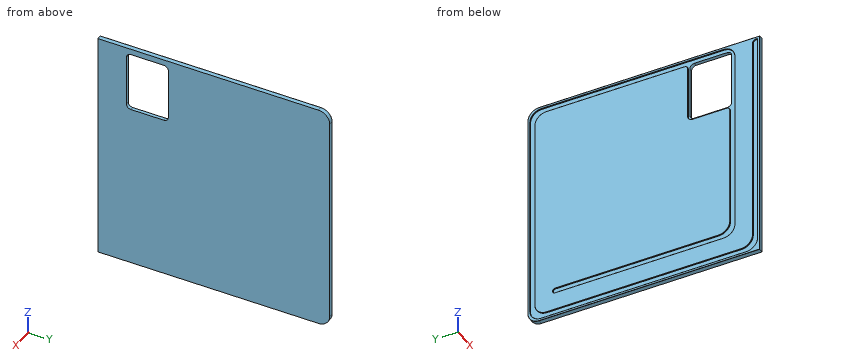
```python
from build123d import *

# Parameters (mm, degrees)
BOSS_EXTRUDE1_DEPTH = 4
CUT_EXTRUDE3_START  = -4
CUT_EXTRUDE3_DEPTH  = 1
FILLET1_R           = 0.2
CUT_EXTRUDE4_REACH  = 146.305


with BuildPart() as part:
    # Sketch1 → Boss-Extrude1 (new body)
    with BuildSketch(Plane(origin=(0, 0, 0), x_dir=(0, 0, -1), z_dir=(1, 0, 0))):
        with BuildLine():
            Line((-102, -102), (102, -102))
            Line((102, -102), (102, 92))
            ThreePointArc((102, 92), (99.071067812, 99.071067812), (92, 102))
            Line((92, 102), (-92, 102))
            ThreePointArc((-92, 102), (-99.071067812, 99.071067812), (-102, 92))
            Line((-102, 92), (-102, -102))
        make_face()
    extrude(amount=BOSS_EXTRUDE1_DEPTH)

    # Sketch2 → Cut-Extrude3 (cut)
    with BuildSketch(Plane(origin=(4, 0, 0), x_dir=(0, 0, -1), z_dir=(1, 0, 0)).offset(CUT_EXTRUDE3_START)):
        with BuildLine():
            Line((-100.1, 90.3), (-100.1, -70.3))
            ThreePointArc((-100.1, -70.3), (-97.229646456, -77.229646456), (-90.3, -80.1))
            Line((-90.3, -80.1), (70.3, -80.1))
            ThreePointArc((70.3, -80.1), (77.229646456, -77.229646456), (80.1, -70.3))
            Line((80.1, -70.3), (80.1, 78))
            ThreePointArc((80.1, 78), (78, 80.1), (75.9, 78))
            Line((75.9, 78), (75.9, -65.7))
            ThreePointArc((75.9, -65.7), (72.912489168, -72.912489168), (65.7, -75.9))
            Line((65.7, -75.9), (-40.2, -75.9))
            ThreePointArc((-40.2, -75.9), (-42.321320344, -75.021320344), (-43.2, -72.9))
            Line((-43.2, -72.9), (-43.2, -42.8))
            ThreePointArc((-43.2, -42.8), (-44.371572875, -39.971572875), (-47.2, -38.8))
            Line((-47.2, -38.8), (-92.9, -38.8))
            ThreePointArc((-92.9, -38.8), (-95.021320344, -37.921320344), (-95.9, -35.8))
            Line((-95.9, -35.8), (-95.9, 85.7))
            ThreePointArc((-95.9, 85.7), (-92.912489168, 92.912489168), (-85.7, 95.9))
            Line((-85.7, 95.9), (85.7, 95.9))
            ThreePointArc((85.7, 95.9), (92.912489168, 92.912489168), (95.9, 85.7))
            Line((95.9, 85.7), (95.9, -85.7))
            ThreePointArc((95.9, -85.7), (92.912489168, -92.912489168), (85.7, -95.9))
            Line((85.7, -95.9), (-97.3, -95.9))
            ThreePointArc((-97.3, -95.9), (-99.279898987, -96.720101013), (-100.1, -98.7))
            Line((-100.1, -98.7), (-100.1, -100.1))
            Line((-100.1, -100.1), (90.3, -100.1))
            ThreePointArc((90.3, -100.1), (97.229646456, -97.229646456), (100.1, -90.3))
            Line((100.1, -90.3), (100.1, 90.3))
            ThreePointArc((100.1, 90.3), (97.229646456, 97.229646456), (90.3, 100.1))
            Line((90.3, 100.1), (-90.3, 100.1))
            ThreePointArc((-90.3, 100.1), (-97.229646456, 97.229646456), (-100.1, 90.3))
        make_face()
        with BuildLine():
            Line((-90.9, -75.9), (-48.4, -75.9))
            ThreePointArc((-48.4, -75.9), (-46.278679656, -75.021320344), (-45.4, -72.9))
            Line((-45.4, -72.9), (-45.4, -65.9))
            Line((-45.4, -65.9), (-46.4, -65.9))
            Line((-46.4, -65.9), (-46.4, -64.4))
            Line((-46.4, -64.4), (-45.4, -64.4))
            Line((-45.4, -64.4), (-45.4, -62.5))
            Line((-45.4, -62.5), (-46.4, -62.5))
            Line((-46.4, -62.5), (-46.4, -61))
            Line((-46.4, -61), (-45.4, -61))
            Line((-45.4, -61), (-45.4, -45))
            ThreePointArc((-45.4, -45), (-46.571572875, -42.171572875), (-49.4, -41))
            Line((-49.4, -41), (-92.9, -41))
            ThreePointArc((-92.9, -41), (-95.021320344, -41.878679656), (-95.9, -44))
            Line((-95.9, -44), (-95.9, -61))
            Line((-95.9, -61), (-94.9, -61))
            Line((-94.9, -61), (-94.9, -62.5))
            Line((-94.9, -62.5), (-95.9, -62.5))
            Line((-95.9, -62.5), (-95.9, -64.4))
            Line((-95.9, -64.4), (-94.9, -64.4))
            Line((-94.9, -64.4), (-94.9, -65.9))
            Line((-94.9, -65.9), (-95.9, -65.9))
            Line((-95.9, -65.9), (-95.9, -70.9))
            ThreePointArc((-95.9, -70.9), (-94.435533906, -74.435533906), (-90.9, -75.9))
        make_face(mode=Mode.SUBTRACT)
    extrude(amount=CUT_EXTRUDE3_DEPTH, mode=Mode.SUBTRACT)

    # Fillet1
    fillet1_edges = [part.edges().sort_by_distance(p)[0] for p in [
        (0, -72.912489168, -72.912489168),
        (0, -75.021320344, 42.321320344),
        (0, -37.921320344, 95.021320344),
        (0, 92.912489168, 92.912489168),
        (0, 92.912489168, -92.912489168),
        (0, -92.912489168, -92.912489168),
        (0, -96.720101013, 99.279898987),
        (0, -95.9, 5.8),
        (0, 0, -95.9),
        (0, 95.9, 0),
        (0, 24.95, 95.9),
        (0, -38.8, 70.05),
        (0, -39.971572875, 44.371572875),
        (0, -57.85, 43.2),
        (0, -75.9, -12.75),
        (0, 6.15, -75.9),
        (0, 80.1, -78),
        (0, 3.85, -80.1),
        (0, -77.229646456, -77.229646456),
        (0, -80.1, 10),
        (0, -77.229646456, 97.229646456),
        (0, 10, 100.1),
        (0, 97.229646456, 97.229646456),
        (0, 100.1, 0),
        (0, 97.229646456, -97.229646456),
        (0, -102, 0),
        (0, 0, -100.1),
        (0, -97.229646456, -97.229646456),
        (0, -100.1, 4.9),
        (0, -99.4, 100.1),
        (0, -65.15, 94.9),
        (0, -65.9, 95.4),
        (0, -68.4, 95.9),
        (0, -74.435533906, 94.435533906),
        (0, -75.9, 69.65),
        (0, -75.021320344, 46.278679656),
        (0, -69.4, 45.4),
        (0, -5, 102),
        (0, -65.9, 45.9),
        (0, -65.15, 46.4),
        (0, -64.4, 45.9),
        (0, -63.45, 45.4),
        (0, -62.5, 45.9),
        (0, -61.75, 46.4),
        (0, -61, 45.9),
        (0, -53, 45.4),
        (0, -42.171572875, 46.571572875),
        (0, -41, 71.15),
        (0, 99.071067812, 99.071067812),
        (0, -41.878679656, 95.021320344),
        (0, -52.5, 95.9),
        (0, -61, 95.4),
        (0, -61.75, 94.9),
        (0, -62.5, 95.4),
        (0, -63.45, 95.9),
        (0, -64.4, 95.4),
        (0, 102, 0),
        (0, 99.071067812, -99.071067812),
        (0, -5, -102),
    ]]
    fillet(fillet1_edges, radius=FILLET1_R)

    # Sketch4 → Cut-Extrude4 (cut, up to next)
    with BuildSketch(Plane(origin=(4, 0, 0), x_dir=(0, 0, -1), z_dir=(1, 0, 0)), mode=Mode.PRIVATE) as cut_extrude4_sk1:
        with BuildLine():
            Line((-92.9, -40), (-48.4, -40))
            ThreePointArc((-48.4, -40), (-45.571572875, -41.171572875), (-44.4, -44))
            Line((-44.4, -44), (-44.4, -72.9))
            ThreePointArc((-44.4, -72.9), (-45.571572875, -75.728427125), (-48.4, -76.9))
            Line((-48.4, -76.9), (-92.9, -76.9))
            ThreePointArc((-92.9, -76.9), (-95.728427125, -75.728427125), (-96.9, -72.9))
            Line((-96.9, -72.9), (-96.9, -44))
            ThreePointArc((-96.9, -44), (-95.728427125, -41.171572875), (-92.9, -40))
        make_face()
    cut_extrude4_tool1 = extrude(cut_extrude4_sk1.sketch, amount=-CUT_EXTRUDE4_REACH, mode=Mode.PRIVATE) & part.part
    add(cut_extrude4_tool1.solids().sort_by_distance((4, -58.45, 70.65))[0], mode=Mode.SUBTRACT)


solid = part.part
```
Model file for the job. Use its own axes, mm. Give positions to 0.01 mm unless a question says otherwise; leave off trailing zeros. Loops run counter-clockwise (first coordinate to the right, second up) from the corner with the lowest first, then second, coordinate; pieces in that order, holes last. Notation, with made-up numbers: (31, 64) -> (90, 64) arc R35 ccw to (90, 97) -> close; hole circle Ø8 at (40.25, 49.25). An arc over 180 degrees is marked (long way). Use CSV: the item, a comma, the result in double quotes. Start each with the question number.
1) Wall check: line 1 (Z direction, x = 0.4, y = -7); line 2 (Z direction, x = 1.05, y = -56). Give the ranges that are in metal, low to high.
2) Slice it at B-B on x = 1.7. Give the cut face in (y, z), plus the area to 3 significant figures.
3) Slice it at C-C on z = -31. Give the cut face in (x, y).
4) Slice it at A-A on y = -58. Give the cut face in (x, z), plus the area to 3 significant figures.
Computed values:
1,line 1,"z = -102 to -100.1, -95.9 to -80.1, -75.9 to 95.9, 100.1 to 102"
1,line 2,"z = -102 to 44.4, 96.9 to 102"
2,outline,"(-102, -102) -> (92, -102) arc R10 ccw to (102, -92) -> (102, 92) arc R10 ccw to (92, 102) -> (-102, 102) -> close; hole (-76.9, 48.4) arc R4 ccw to (-72.9, 44.4) -> (-44, 44.4) arc R4 ccw to (-40, 48.4) -> (-40, 92.9) arc R4 ccw to (-44, 96.9) -> (-72.9, 96.9) arc R4 ccw to (-76.9, 92.9) -> close"
2,area,"39,600 mm^2"
3,outline,"(0, -101.8) arc R0.2 ccw to (0.2, -102) -> (4, -102) -> (4, 102) -> (0.2, 102) arc R0.2 ccw to (0, 101.8) -> (0, 100.3) arc R0.2 ccw to (0.2, 100.1) -> (1, 100.1) -> (1, 95.9) -> (0.2, 95.9) arc R0.2 ccw to (0, 95.7) -> (0, -75.7) arc R0.2 ccw to (0.2, -75.9) -> (1, -75.9) -> (1, -80.1) -> (0.2, -80.1) arc R0.2 ccw to (0, -80.3) -> (0, -95.7) arc R0.2 ccw to (0.2, -95.9) -> (1, -95.9) -> (1, -100.1) -> (0.2, -100.1) arc R0.2 ccw to (0, -100.3) -> close"
4,outline,"(0, -101.8) arc R0.2 ccw to (0.2, -102) -> (4, -102) -> (4, 44.4) -> (1, 44.4) -> (1, 43.2) -> (0.2, 43.2) arc R0.2 ccw to (0, 43) -> (0, -75.7) arc R0.2 ccw to (0.2, -75.9) -> (1, -75.9) -> (1, -80.1) -> (0.2, -80.1) arc R0.2 ccw to (0, -80.3) -> (0, -95.7) arc R0.2 ccw to (0.2, -95.9) -> (1, -95.9) -> (1, -100.1) -> (0.2, -100.1) arc R0.2 ccw to (0, -100.3) -> close; (0, 100.3) arc R0.2 ccw to (0.2, 100.1) -> (1, 100.1) -> (1, 96.9) -> (4, 96.9) -> (4, 102) -> (0.2, 102) arc R0.2 ccw to (0, 101.8) -> close"
4,area,"593 mm^2"
